Could you check a few things on this drawing? It's one solid part, dimensions in mm from its lowest x, y, z. Give positions to 0.01 mm unless a question says otherwise; leave off trailing zeros. Order: outer loops, then holes, each group sorted by start corner. A loop starts at its lowest first (then second) coordinate and runs counter-clockwise, first axis right, second up. Notation, with made-up numbers: (63, -21.5) -> (89, -21.5) arc R24 cw to (89, 12.5) -> close; hole circle Ø3 at (70, -4.5). An arc over 180 degrees is marked (long way). Write each question's results on one line, items separated by ' | '. Start each with the question number.
Q1. I need wall thicknesses on line 1 along X through (y, z) = (1, 4); line 2 along Z through (x, y) = (7.25, 4.5); line 3 along Y through (x, z) = (0.5, 6.75). Which ranges of each line are inside material? Lowest first, please. Write a range as [from, to].
Q2. Imagine slicing it at C-C, the plane z = 2.75. Please give me the cut outline in (x, y).
Q3. I'm going to push flat-ended pins straight in: pin 1 (3 mm diameter, centred on y = 6.5, z = 6, fed in from -X); pin 2 (1 mm diameter, centred on y = 5, z = 1.5, fed in from +X); pin 3 (2 mm diameter, centred on x = 6.5, z = 6.5, fed in from -Y). Where does each tip first touch, or does it pass through?
Q4. Imagine slicing it at D-D, the plane z = 7. Please give me the cut outline in (x, y), then the cut area to 3 significant figures.
Q5. Imagine slicing it at A-A, the plane y = 3.8. Please give me the cut outline in (x, z), then the cut area to 3 significant figures.
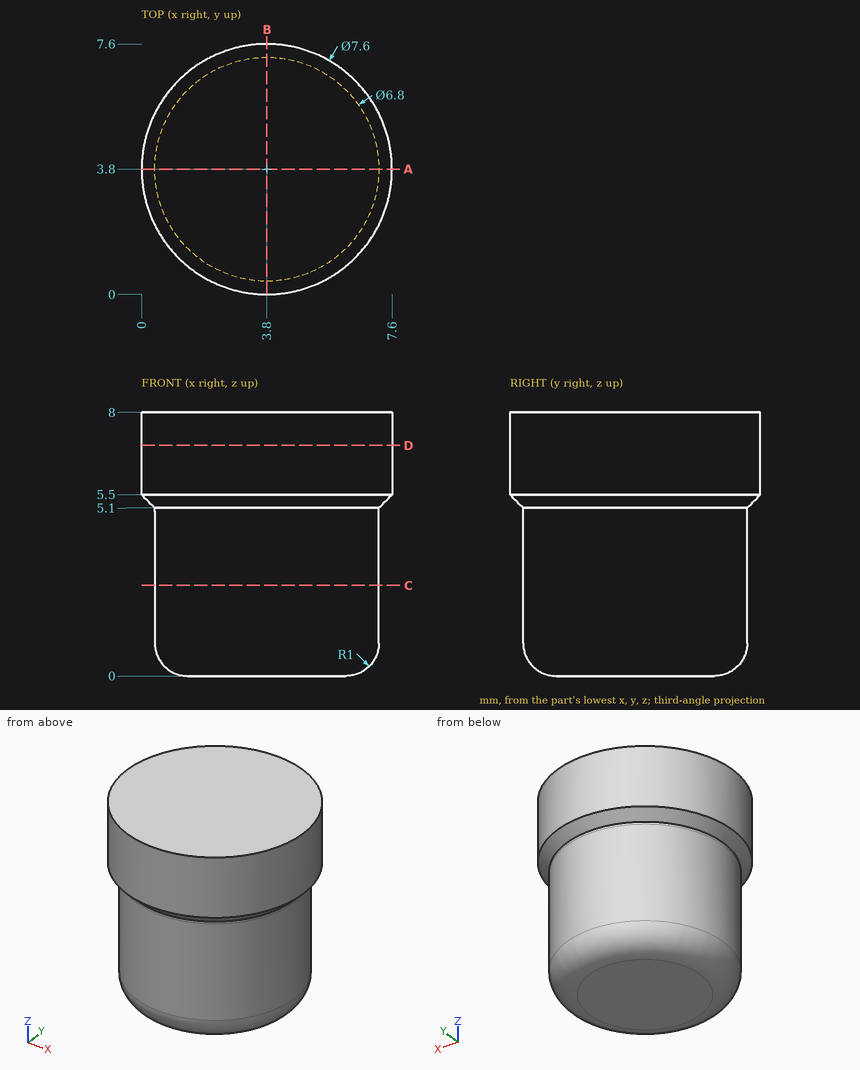
Geometry check:
1) line 1: [1.87, 5.73] | line 2: [5.22, 8] | line 3: [1.92, 5.68]
2) outline: circle Ø6.8 at (3.8, 3.8)
3) pin 1: x = 0.19 | pin 2: x = 7.13 | pin 3: y = 0.4
4) outline: circle Ø7.6 at (3.8, 3.8) | area: 45.4 mm²
5) outline: (0, 5.5) -> (0.4, 5.1) -> (0.4, 1) arc R1 ccw to (1.4, 0) -> (6.2, 0) arc R1 ccw to (7.2, 1) -> (7.2, 5.1) -> (7.6, 5.5) -> (7.6, 8) -> (0, 8) -> close | area: 56.1 mm²
